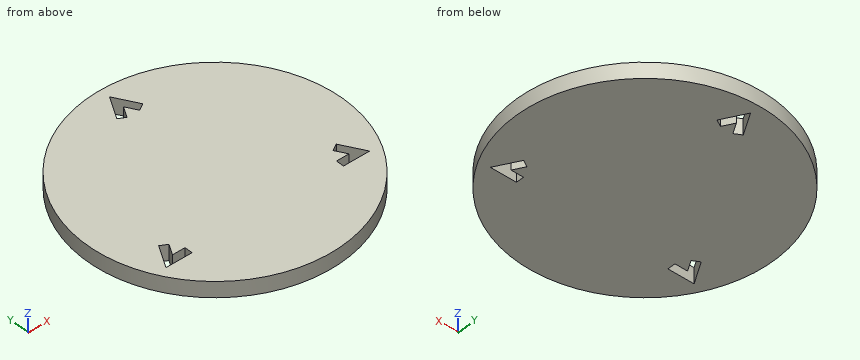
from build123d import *

# Parameters (mm, degrees)
CROQUIS1_R              = 49
SALIENTE_EXTRUIR1_DEPTH = 6


with BuildPart() as part:
    # Croquis1 → Saliente-Extruir1 (new body)
    # profile 1 of 2: a face of its own
    with BuildSketch(Plane.XY):
        Circle(CROQUIS1_R)
        Polygon((-5, 36.339745962), (0, 45), (5, 36.339745962), (33.97114317, -13.839745962), (38.97114317, -22.5), (28.97114317, -22.5), (-28.97114317, -22.5), (-38.97114317, -22.5), (-33.97114317, -13.839745962), align=None, mode=Mode.SUBTRACT)
    # profile 2 of 2: a face of its own
    with BuildSketch(Plane.XY):
        Polygon((-2.401923789, 34.839745962), (-5, 36.339745962), (-33.97114317, -13.839745962), (-31.373066959, -15.339745962), (-33.774990748, -19.5), (-28.97114317, -19.5), (-28.97114317, -22.5), (28.97114317, -22.5), (28.97114317, -19.5), (33.774990748, -19.5), (31.373066959, -15.339745962), (33.97114317, -13.839745962), (5, 36.339745962), (2.401923789, 34.839745962), (0, 39), align=None)
    extrude(amount=SALIENTE_EXTRUIR1_DEPTH)


solid = part.part
Build history of the part. All positions in model axes, mm. Round coordinates to 2 decimals unless told otherwise and drop trailing zeros. Order: outer loops, then holes, each group sorted by start corner. A loop starts at its lowest first (then second) coordinate and runs counter-clockwise, first axis right, second up. Notation, with made-up numbers: M -3.75,10.5 L 24.25,10.5 A20 ccw 24.25,42.5 Z; hole C 20.25,72.25 d9. An arc over 180 degrees is marked long. Use CSV: the item, a comma, the result in double quotes. Start each with the question number.
(1) Flat gauge pins, fed straight in: P1, Ø2.5, axis at x = 30.5, z = 4.5, coming from the -Y side; P2, Ø3.5, axis at y = -21, z = 4, coming from the +X side; P3, Ø0.9, axis at y = -21.5, z = 2, coming from the -X side. Where does each tip first touch, or does it go through?
(2) Cut at C-C on x = 12. List the corners of the cut face in (y, z).
(3) Cut at A-A on z = 2.75. List the corners of the cut face in (x, y) (3 decimals).
(4) Drill centre lines: probe 1 along Y at (x, z) = (4, 2); probe 2 along Y at (x, z) = (39.5, 5.5); probe 3 along X at (y, z) = (-18, 2.15). Where is each one in solid material? Low to high.
(5) Cut at B-B on y = 16.5. List the corners of the cut face in (x, z).
Findings:
1,P1,"stops at y = -39.31"
1,P2,"stops at x = 45.06"
1,P3,"stops at x = -44.25"
2,outline,"M -47.51,0 L 47.51,0 L 47.51,6 L -47.51,6 Z"
3,outline,"C 0,0 d98; hole M -38.971,-22.5 L -28.971,-22.5 L -28.971,-19.5 L -33.775,-19.5 L -31.373,-15.34 L -33.971,-13.84 Z; hole M -5,36.34 L -2.402,34.84 L 0,39 L 2.402,34.84 L 5,36.34 L 0,45 Z; hole M 28.971,-22.5 L 38.971,-22.5 L 33.971,-13.84 L 31.373,-15.34 L 33.775,-19.5 L 28.971,-19.5 Z"
4,probe 1,"y = -48.84 to 35.76, 38.07 to 48.84"
4,probe 2,"y = -29 to 29"
4,probe 3,"x = -45.57 to -36.37, -32.91 to 32.91, 36.37 to 45.57"
5,outline,"M -46.14,0 L 46.14,0 L 46.14,6 L -46.14,6 Z"
